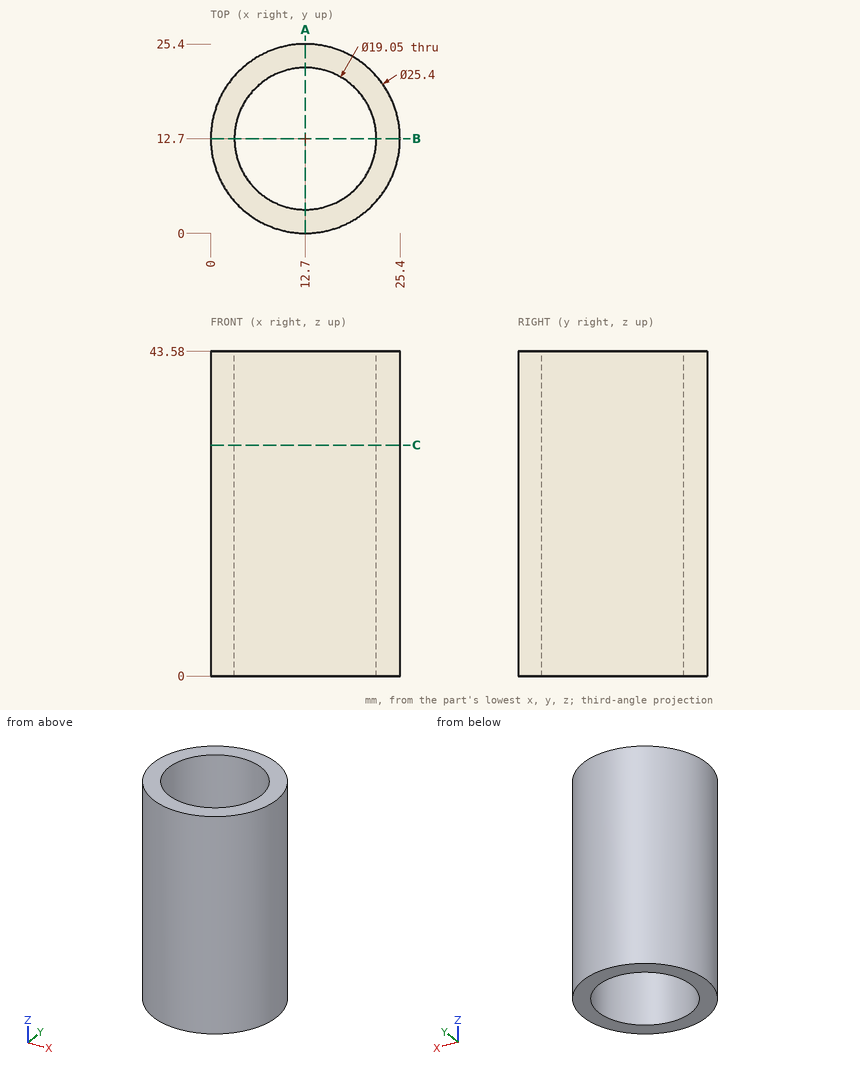
Job drawing, mm, ordinate dimensions from the low corner. One solid piece. Coordinates: 2 decimals unless noted, no trailing zeros. Order: outer loops, then holes, each group sorted by start corner. A loop starts at its lowest first (then second) coordinate and runs counter-clockwise, first axis right, second up. Notation, with made-up numbers: (19, 77) -> (45, 77) arc R25 ccw to (45, 106) -> close; hole circle Ø4 at (77.5, 9.25). An arc over 180 degrees is marked (long way). Put each result on its own line as item: value. Start each with the question number.
(1) Band-saw the part on C-C (z = 31). Give the cut face in (x, y) (3 decimals).
(2) Probe line 1 along X through (y, z) = (17.75, 3.5); line 2 along X through (y, z) = (16.75, 37); line 3 along Y through (x, z) = (5.5, 29). List the from-to ranges inside material, lowest first. Write a range as [from, to].
(3) Band-saw the part on A-A (x = 12.7). Give the cut face in (y, z) (3 decimals).
(4) Pin check, flat tips, straight feed: pin 1 Ø5 at (x, z) = (5.5, 26) entering from -Y; pin 2 Ø1.5 at (y, z) = (4.5, 24.5) entering from -X. Stop position of each tip, or through.
Determined:
1. outline: circle Ø25.4 at (12.7, 12.7); hole circle Ø19.05 at (12.7, 12.7)
2. line 1: x = [1.05, 4.62], [20.78, 24.35]
2. line 2: x = [0.66, 4.08], [21.32, 24.74]
2. line 3: y = [2.24, 6.46], [18.94, 23.16]
3. outline: (0, 0) -> (3.175, 0) -> (3.175, 43.58) -> (0, 43.58) -> close; (22.225, 0) -> (25.4, 0) -> (25.4, 43.58) -> (22.225, 43.58) -> close
4. pin 1: stops at y = 0.9
4. pin 2: stops at x = 2.41
